The figure shows three views and two pictorial views of one solid part (mm, origin at its lowest corner). Answer the questions. A direction names the side the tool comes from. Coordinates: 2 decimals unless noted, no trailing zeros. Loops run counter-clockwise (first coordinate to the right, second up) from the corner with the lowest first, then second, coordinate; pieces in that order, holes last.
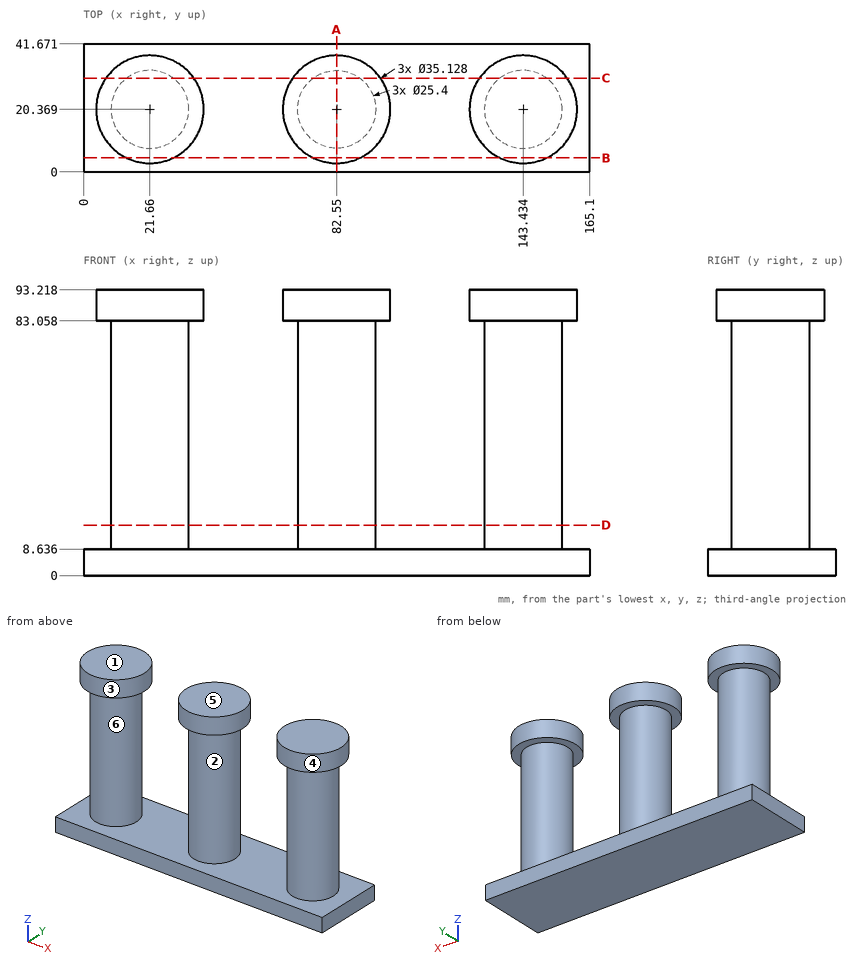
Q1. Determine the mould class of the marked faces 1, 2 and 3 for opening direction X: +X half, -X half, draft (parallel to the pull), parting line (faces both ways), or undercut.
Findings below:
face 1: draft
face 2: undercut
face 3: undercut
Q2. A cutting plane is placed at D-D (z = 16.5). Give the vertices of the cut face in (x, y), then the cut area to 3 significant figures.
Findings below:
outline: circle Ø25.4 at (21.66, 20.37); circle Ø25.4 at (82.55, 20.37); circle Ø25.4 at (143.43, 20.37)
area: 1,520 mm2
Q3. Flat-ended cylindrical pins translate along their axes: pin 1 Ø5 at (x, z) = (20, 81.5) entering from -Y (1 decimal); pin 2 Ø21 at (x, y) = (59, 16.5) entering from +Z; pin 3 Ø6 at (y, z) = (26.5, 29) entering from +X; pin 4 Ø1.5 at (x, z) = (93, 62.5) entering from -Y. Find the tip coordinate at first contact, or state that the pin passes through.
Findings below:
pin 1: stops at y = 2.8
pin 2: stops at z = 93.22
pin 3: stops at x = 155.74
pin 4: stops at y = 12.17
Q4. A cutting plane is placed at A-A (x = 82.55). Give the vertices of the cut face in (y, z) (1 decimal), then the cut area to 3 significant figures.
Findings below:
outline: (0, 0) - (41.7, 0) - (41.7, 8.6) - (33.1, 8.6) - (33.1, 83.1) - (37.9, 83.1) - (37.9, 93.2) - (2.8, 93.2) - (2.8, 83.1) - (7.7, 83.1) - (7.7, 8.6) - (0, 8.6) - close
area: 2,610 mm2
Q5. Straight lines are drawn through the part: probe 1 along Z at (x, y) = (130, 17); probe 2 along X at (y, z) = (16.5, 23) (1 decimal); probe 3 along X at (y, z) = (21.5, 60.5) (1 decimal). For each, find the intervals that lie inside material, in ascending order.
Findings below:
probe 1: z = 0 to 8.64, 83.06 to 93.22
probe 2: x = 9.6 to 33.8, 70.5 to 94.6, 131.3 to 155.5
probe 3: x = 9 to 34.3, 69.9 to 95.2, 130.8 to 156.1
Q6. A cutting plane is placed at B-B (y = 4.5). Give the vertices of the cut face in (x, z) (1 decimal).
Findings below:
outline: (0, 0) - (165.1, 0) - (165.1, 8.6) - (0, 8.6) - close; (14.1, 83.1) - (29.2, 83.1) - (29.2, 93.2) - (14.1, 93.2) - close; (75, 83.1) - (90.1, 83.1) - (90.1, 93.2) - (75, 93.2) - close; (135.9, 83.1) - (151, 83.1) - (151, 93.2) - (135.9, 93.2) - close
Q7. A cutting plane is placed at C-C (y = 30.5). Give the vertices of the cut face in (x, z) (1 decimal).
Findings below:
outline: (0, 0) - (165.1, 0) - (165.1, 8.6) - (151.1, 8.6) - (151.1, 83.1) - (157.8, 83.1) - (157.8, 93.2) - (129.1, 93.2) - (129.1, 83.1) - (135.8, 83.1) - (135.8, 8.6) - (90.2, 8.6) - (90.2, 83.1) - (96.9, 83.1) - (96.9, 93.2) - (68.2, 93.2) - (68.2, 83.1) - (74.9, 83.1) - (74.9, 8.6) - (29.3, 8.6) - (29.3, 83.1) - (36, 83.1) - (36, 93.2) - (7.3, 93.2) - (7.3, 83.1) - (14, 83.1) - (14, 8.6) - (0, 8.6) - close
Q8. Which of the six approach directions +Z, -Z, +X, -X, +Y, -Y give full straight-line access (tool end or side, diameter ignored) to the marked faces 4, 5 and 6?
Findings below:
face 4: +Z
face 5: +Z, +X, -X, +Y, -Y
face 6: none
